Geometry: see drawing. Coordinates: mm, zero at the bounding-box minimum. A direction names the side the tool comes from. Coordinates: 2 decimals unless noted, no trailing zeros. Write each loop counter-clockwise with the first axis right and the second up, starting at its lowest first coordinate (ties: lowest second). Pieces come first, ordered by that corner, then holes.
1) Section query A-A (y = 8). Output: boundary loops of the cut face in (x, z) (1 decimal).
2) Pin query (flat end, axial travel): pin 1 Ø6 at (y, z) = (42.5, 57.5) entering from +X; pin 2 Ø1 at (y, z) = (34, 37) entering from +X; pin 3 Ø5 at (y, z) = (35.5, 26) entering from -X; pin 4 Ø9 at (x, z) = (34.5, 21) entering from -Y. Return the tip coordinate at first contact, or that it passes through.
3) Line query: L1, parallel to X at y = 30, z = 29; L2, parallel to Z at x = 47.5, y = 25.5; L3, parallel to X at y = 33, z = 40. Output: solid intervals per line, ascending.
4) Section query B-B (z = 21). Output: boundary loops of the cut face in (x, y) (1 decimal).
5) Set-up query: the marked faces 1, 2 and 3. Return all of +Z, -Z, +X, -X, +Y, -Y with unobstructed straight access to the full face (end or side cutting, diameter ignored); none if empty.
6) Section query D-D (x = 26.5). Output: boundary loops of the cut face in (y, z) (1 decimal).
7) Draft query along X for the marked faces 4, 5 and 6. Return one class per face: pulls with the +X half, pulls with the -X half, needs draft (parallel to the pull), parting line crosses it, or undercut.
8) Section query C-C (y = 36). Output: boundary loops of the cut face in (x, z) (1 decimal), then the cut area to 3 significant figures.
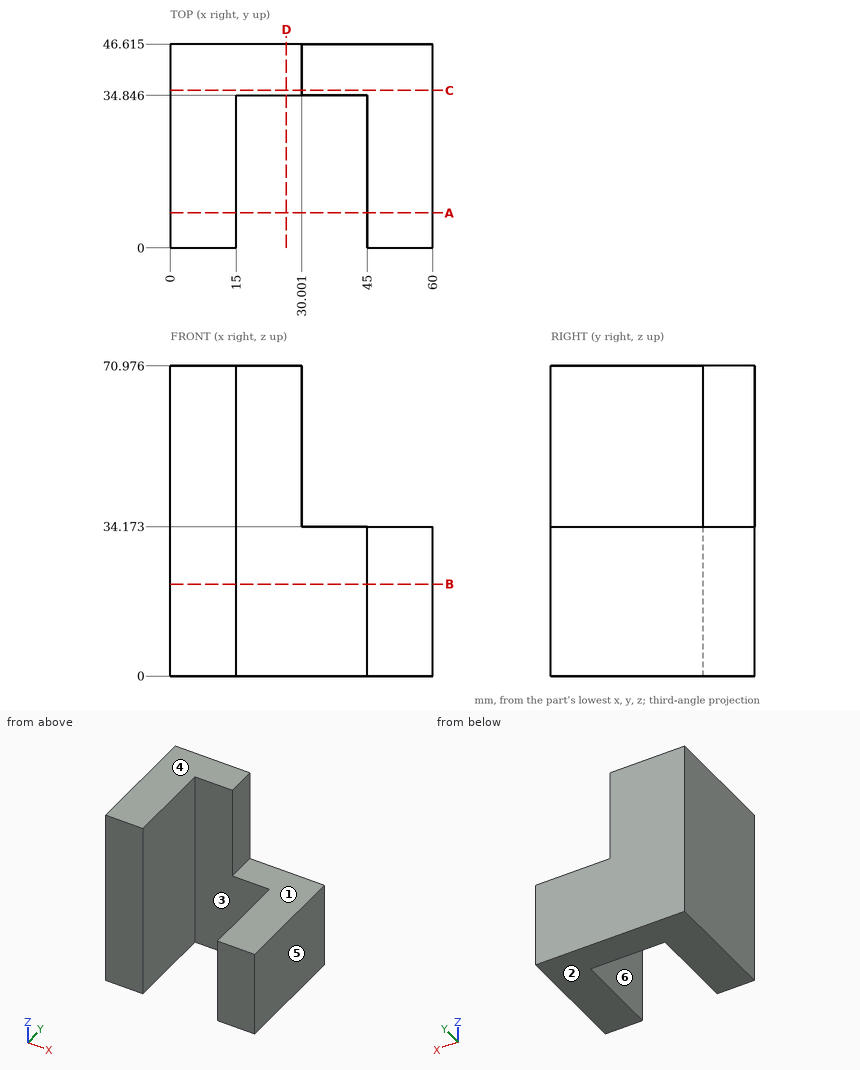
Answer:
1. outline: (0, 0) - (15, 0) - (15, 71) - (0, 71) - close; (45, 0) - (60, 0) - (60, 34.2) - (45, 34.2) - close
2. pin 1: stops at x = 30
2. pin 2: stops at x = 15
2. pin 3: stops at x = 0
2. pin 4: stops at y = 34.85
3. L1: x = 0 to 15, 45 to 60
3. L2: z = 0 to 34.17
3. L3: x = 0 to 15
4. outline: (0, 0) - (15, 0) - (15, 34.8) - (45, 34.8) - (45, 0) - (60, 0) - (60, 46.6) - (0, 46.6) - close
5. face 1: +Z, +X, +Y, -Y
5. face 2: -Z, +X, -X, +Y, -Y
5. face 3: +Z, -Z, -Y
6. outline: (34.8, 0) - (46.6, 0) - (46.6, 71) - (34.8, 71) - close
7. face 4: needs draft
7. face 5: pulls with the +X half
7. face 6: undercut
8. outline: (0, 0) - (60, 0) - (60, 34.2) - (30, 34.2) - (30, 71) - (0, 71) - close
8. area: 3,150 mm2
